```python
from build123d import *

# Parameters (mm, degrees)
ESQUISSE1_W             = 15.25
ESQUISSE1_H             = 174
BOSS_EXTRU_1_DEPTH      = 300
ESQUISSE2_W             = 15.25
ESQUISSE2_H             = 28.357142857
BOSS_EXTRU_2_DEPTH      = 15.25
ENL_V_MAT_EXTRU_1_REACH = 17.25
ESQUISSE3_R             = 4


with BuildPart() as part:
    # Esquisse1 → Boss.-Extru.1 (new body)
    with BuildSketch(Plane.XY):
        with Locations((457.625, 83.063864629)):
            Rectangle(ESQUISSE1_W, ESQUISSE1_H)
    extrude(amount=BOSS_EXTRU_1_DEPTH)

    # Esquisse2 → Boss.-Extru.2 (add)
    with BuildSketch(Plane(origin=(465.25, 0, 0), x_dir=(0, 0, -1), z_dir=(1, 0, 0))):
        with Locations((7.625, 141.278150344)):
            Rectangle(ESQUISSE2_W, ESQUISSE2_H)
        with Locations((7.625, 82.563864628)):
            Rectangle(ESQUISSE2_W, ESQUISSE2_H)
        with Locations((7.625, 23.849578915)):
            Rectangle(ESQUISSE2_W, ESQUISSE2_H)
    extrude(amount=-BOSS_EXTRU_2_DEPTH)

    # Esquisse3 → Enlèv. mat.-Extru.1 (cut, up to next)
    with BuildSketch(Plane(origin=(465.25, 0, 0), x_dir=(0, 0, -1), z_dir=(1, 0, 0)), mode=Mode.PRIVATE) as enl_v_mat_extru_1_sk1:
        with Locations((-110, 145.456721772)):
            Circle(ESQUISSE3_R)
    enl_v_mat_extru_1_tool1 = extrude(enl_v_mat_extru_1_sk1.sketch, amount=-ENL_V_MAT_EXTRU_1_REACH, mode=Mode.PRIVATE) & part.part
    add(enl_v_mat_extru_1_tool1.solids().sort_by_distance((465.25, 145.456722, 110))[0], mode=Mode.SUBTRACT)
    # Esquisse3 → Enlèv. mat.-Extru.1 (cut, up to next)
    with BuildSketch(Plane(origin=(465.25, 0, 0), x_dir=(0, 0, -1), z_dir=(1, 0, 0)), mode=Mode.PRIVATE) as enl_v_mat_extru_1_sk2:
        with Locations((-110, 70.456721772)):
            Circle(ESQUISSE3_R)
    enl_v_mat_extru_1_tool2 = extrude(enl_v_mat_extru_1_sk2.sketch, amount=-ENL_V_MAT_EXTRU_1_REACH, mode=Mode.PRIVATE) & part.part
    add(enl_v_mat_extru_1_tool2.solids().sort_by_distance((465.25, 70.456722, 110))[0], mode=Mode.SUBTRACT)
    # Esquisse3 → Enlèv. mat.-Extru.1 (cut, up to next)
    with BuildSketch(Plane(origin=(465.25, 0, 0), x_dir=(0, 0, -1), z_dir=(1, 0, 0)), mode=Mode.PRIVATE) as enl_v_mat_extru_1_sk3:
        with Locations((-150, 70.456721772)):
            Circle(ESQUISSE3_R)
    enl_v_mat_extru_1_tool3 = extrude(enl_v_mat_extru_1_sk3.sketch, amount=-ENL_V_MAT_EXTRU_1_REACH, mode=Mode.PRIVATE) & part.part
    add(enl_v_mat_extru_1_tool3.solids().sort_by_distance((465.25, 70.456722, 150))[0], mode=Mode.SUBTRACT)
    # Esquisse3 → Enlèv. mat.-Extru.1 (cut, up to next)
    with BuildSketch(Plane(origin=(465.25, 0, 0), x_dir=(0, 0, -1), z_dir=(1, 0, 0)), mode=Mode.PRIVATE) as enl_v_mat_extru_1_sk4:
        with Locations((-150, 145.456721772)):
            Circle(ESQUISSE3_R)
    enl_v_mat_extru_1_tool4 = extrude(enl_v_mat_extru_1_sk4.sketch, amount=-ENL_V_MAT_EXTRU_1_REACH, mode=Mode.PRIVATE) & part.part
    add(enl_v_mat_extru_1_tool4.solids().sort_by_distance((465.25, 145.456722, 150))[0], mode=Mode.SUBTRACT)
    # Esquisse3 → Enlèv. mat.-Extru.1 (cut, up to next)
    with BuildSketch(Plane(origin=(465.25, 0, 0), x_dir=(0, 0, -1), z_dir=(1, 0, 0)), mode=Mode.PRIVATE) as enl_v_mat_extru_1_sk5:
        with Locations((-190, 145.456721772)):
            Circle(ESQUISSE3_R)
    enl_v_mat_extru_1_tool5 = extrude(enl_v_mat_extru_1_sk5.sketch, amount=-ENL_V_MAT_EXTRU_1_REACH, mode=Mode.PRIVATE) & part.part
    add(enl_v_mat_extru_1_tool5.solids().sort_by_distance((465.25, 145.456722, 190))[0], mode=Mode.SUBTRACT)
    # Esquisse3 → Enlèv. mat.-Extru.1 (cut, up to next)
    with BuildSketch(Plane(origin=(465.25, 0, 0), x_dir=(0, 0, -1), z_dir=(1, 0, 0)), mode=Mode.PRIVATE) as enl_v_mat_extru_1_sk6:
        with Locations((-190, 70.456721772)):
            Circle(ESQUISSE3_R)
    enl_v_mat_extru_1_tool6 = extrude(enl_v_mat_extru_1_sk6.sketch, amount=-ENL_V_MAT_EXTRU_1_REACH, mode=Mode.PRIVATE) & part.part
    add(enl_v_mat_extru_1_tool6.solids().sort_by_distance((465.25, 70.456722, 190))[0], mode=Mode.SUBTRACT)
    # Esquisse3 → Enlèv. mat.-Extru.1 (cut, up to next)
    with BuildSketch(Plane(origin=(465.25, 0, 0), x_dir=(0, 0, -1), z_dir=(1, 0, 0)), mode=Mode.PRIVATE) as enl_v_mat_extru_1_sk7:
        with Locations((-130, 126.706721772)):
            Circle(ESQUISSE3_R)
    enl_v_mat_extru_1_tool7 = extrude(enl_v_mat_extru_1_sk7.sketch, amount=-ENL_V_MAT_EXTRU_1_REACH, mode=Mode.PRIVATE) & part.part
    add(enl_v_mat_extru_1_tool7.solids().sort_by_distance((465.25, 126.706722, 130))[0], mode=Mode.SUBTRACT)
    # Esquisse3 → Enlèv. mat.-Extru.1 (cut, up to next)
    with BuildSketch(Plane(origin=(465.25, 0, 0), x_dir=(0, 0, -1), z_dir=(1, 0, 0)), mode=Mode.PRIVATE) as enl_v_mat_extru_1_sk8:
        with Locations((-170, 126.706721772)):
            Circle(ESQUISSE3_R)
    enl_v_mat_extru_1_tool8 = extrude(enl_v_mat_extru_1_sk8.sketch, amount=-ENL_V_MAT_EXTRU_1_REACH, mode=Mode.PRIVATE) & part.part
    add(enl_v_mat_extru_1_tool8.solids().sort_by_distance((465.25, 126.706722, 170))[0], mode=Mode.SUBTRACT)
    # Esquisse3 → Enlèv. mat.-Extru.1 (cut, up to next)
    with BuildSketch(Plane(origin=(465.25, 0, 0), x_dir=(0, 0, -1), z_dir=(1, 0, 0)), mode=Mode.PRIVATE) as enl_v_mat_extru_1_sk9:
        with Locations((-190, 107.956721772)):
            Circle(ESQUISSE3_R)
    enl_v_mat_extru_1_tool9 = extrude(enl_v_mat_extru_1_sk9.sketch, amount=-ENL_V_MAT_EXTRU_1_REACH, mode=Mode.PRIVATE) & part.part
    add(enl_v_mat_extru_1_tool9.solids().sort_by_distance((465.25, 107.956722, 190))[0], mode=Mode.SUBTRACT)
    # Esquisse3 → Enlèv. mat.-Extru.1 (cut, up to next)
    with BuildSketch(Plane(origin=(465.25, 0, 0), x_dir=(0, 0, -1), z_dir=(1, 0, 0)), mode=Mode.PRIVATE) as enl_v_mat_extru_1_sk10:
        with Locations((-170, 89.206721772)):
            Circle(ESQUISSE3_R)
    enl_v_mat_extru_1_tool10 = extrude(enl_v_mat_extru_1_sk10.sketch, amount=-ENL_V_MAT_EXTRU_1_REACH, mode=Mode.PRIVATE) & part.part
    add(enl_v_mat_extru_1_tool10.solids().sort_by_distance((465.25, 89.206722, 170))[0], mode=Mode.SUBTRACT)
    # Esquisse3 → Enlèv. mat.-Extru.1 (cut, up to next)
    with BuildSketch(Plane(origin=(465.25, 0, 0), x_dir=(0, 0, -1), z_dir=(1, 0, 0)), mode=Mode.PRIVATE) as enl_v_mat_extru_1_sk11:
        with Locations((-130, 89.206721772)):
            Circle(ESQUISSE3_R)
    enl_v_mat_extru_1_tool11 = extrude(enl_v_mat_extru_1_sk11.sketch, amount=-ENL_V_MAT_EXTRU_1_REACH, mode=Mode.PRIVATE) & part.part
    add(enl_v_mat_extru_1_tool11.solids().sort_by_distance((465.25, 89.206722, 130))[0], mode=Mode.SUBTRACT)
    # Esquisse3 → Enlèv. mat.-Extru.1 (cut, up to next)
    with BuildSketch(Plane(origin=(465.25, 0, 0), x_dir=(0, 0, -1), z_dir=(1, 0, 0)), mode=Mode.PRIVATE) as enl_v_mat_extru_1_sk12:
        with Locations((-110, 107.956721772)):
            Circle(ESQUISSE3_R)
    enl_v_mat_extru_1_tool12 = extrude(enl_v_mat_extru_1_sk12.sketch, amount=-ENL_V_MAT_EXTRU_1_REACH, mode=Mode.PRIVATE) & part.part
    add(enl_v_mat_extru_1_tool12.solids().sort_by_distance((465.25, 107.956722, 110))[0], mode=Mode.SUBTRACT)
    # Esquisse3 → Enlèv. mat.-Extru.1 (cut, up to next)
    with BuildSketch(Plane(origin=(465.25, 0, 0), x_dir=(0, 0, -1), z_dir=(1, 0, 0)), mode=Mode.PRIVATE) as enl_v_mat_extru_1_sk13:
        with Locations((-150, 107.956721772)):
            Circle(ESQUISSE3_R)
    enl_v_mat_extru_1_tool13 = extrude(enl_v_mat_extru_1_sk13.sketch, amount=-ENL_V_MAT_EXTRU_1_REACH, mode=Mode.PRIVATE) & part.part
    add(enl_v_mat_extru_1_tool13.solids().sort_by_distance((465.25, 107.956722, 150))[0], mode=Mode.SUBTRACT)


solid = part.part
```
Model file for the job. Use its own axes, mm. A direction names the side the tool comes from. Give positions to 0.01 mm unless a question says otherwise; leave off trailing zeros. Write each loop counter-clockwise with the first axis right and the second up, starting at its lowest first coordinate (ties: lowest second). Pieces come first, ordered by that corner, then holes. Notation, with made-up numbers: M 74.25,18.25 L 99.25,18.25 A18 ccw 99.25,24.25 Z; hole C 4,75 d2. An arc over 180 degrees is marked long. Use a Markdown table: item, result.
1) Pull direction Z, two halves, no side cores. Call faces 5 (the cylindrical face through (457.73, 111.33, 147.85)), 6 (the flat face through (458, 53, 0)), 7 (the flat face through (458, 38.028, -8)): +Z half, -Z half, draft (parallel to the pull), parting line (faces both ways), or undercut.
Responses:
| item | result |
|---|---|
| face 5 | undercut |
| face 6 | -Z half |
| face 7 | draft |
2) Drill centre lines: line 1 (Y direction, x = 454, z = 150); line 2 (Y direction, x = 456.75, z = 171.5); line 3 (Z direction, x = 456.5, y = 111). Where is each one in solid material? Low to high. Write a range as from..to.
Responses:
| item | result |
|---|---|
| line 1 | y = -3.94..66.46, 74.46..103.96, 111.96..141.46, 149.46..170.06 |
| line 2 | y = -3.94..85.5, 92.91..123, 130.41..170.06 |
| line 3 | z = 0..107.4, 112.6..147.4, 152.6..187.4, 192.6..300 |
3) Tool access for faces 1 (the flat face through (458, 68.385, -8)), 2 (the flat face through (458, 9.671, -8)), 3 (the flat face through (458, 155.457, -8)), 4 (the flat face through (465.25, 82, 140)): list every direction of +Z, -Z, +X, -X, +Y, -Y with a clear straight run to the whole face (end or side of a thin tool).
Responses:
| item | result |
|---|---|
| face 1 | -Z, +X, -X |
| face 2 | -Z, +X, -X, -Y |
| face 3 | -Z, +X, -X, +Y |
| face 4 | +Z, -Z, +X, +Y, -Y |
4) Cut at B-B (x = 461.5). Give the number of separate pieces and of enclosed holes in the cut face, and give its area (3 significant figures).
Responses:
| item | result |
|---|---|
| separate pieces | 1 |
| enclosed holes | 13 |
| area | 52,800 mm2 |
5) Cut at A-A (z = 150). List the corners of the cut face in (x, y), and give its area (3 significant figures).
Responses:
| item | result |
|---|---|
| outline | M 450,-3.94 L 465.25,-3.94 L 465.25,66.46 L 450,66.46 Z; M 450,74.46 L 465.25,74.46 L 465.25,103.96 L 450,103.96 Z; M 450,111.96 L 465.25,111.96 L 465.25,141.46 L 450,141.46 Z; M 450,149.46 L 465.25,149.46 L 465.25,170.06 L 450,170.06 Z |
| area | 2,290 mm2 |
6) Pin check, flat tips, straight feed: pin 1 (7 mm diameter, centred on y = 107.96, z = 110, fed in from +X); pin 2 (1.5 mm diameter, centred on x = 460.5, y = 103.5, fed in from -Z). Stop position of each tip, or through.
Responses:
| item | result |
|---|---|
| pin 1 | passes through |
| pin 2 | stops at z = 0 |
